from build123d import *

# Parameters (mm, degrees)
SKETCH1_W          = 12.7
SKETCH1_H          = 2.413
CHAMFER1_SIZE      = 0.79375
CUT_EXTRUDE2_DEPTH = 1.79578
SKETCH6_R          = 1.833087105
CUT_EXTRUDE3_DEPTH = 1.79578
CUT_EXTRUDE3_TAPER = 45


with BuildPart() as part:
    # Sketch1 → Revolve1 (revolve)
    with BuildSketch(Plane(origin=(0, 0, 0), x_dir=(0, 0, -1), z_dir=(1, 0, 0))):
        with Locations((8.9154, 1.2065)):
            Rectangle(SKETCH1_W, SKETCH1_H)
    revolve(axis=Axis((0, 0, -15.2654), (0, 0, 1)))

    # Chamfer1
    chamfer1_edges = [part.edges().sort_by_distance(p)[0] for p in [
        (0, -2.413, -15.2654),
    ]]
    chamfer(chamfer1_edges, length=CHAMFER1_SIZE)

    # Sketch7 → Revolve2 (revolve)
    with BuildSketch(Plane(origin=(0, 0, 0), x_dir=(0, 0, -1), z_dir=(1, 0, 0)), mode=Mode.PRIVATE) as revolve2_sk:
        with BuildLine():
            Line((2.18059, 4.5847), (2.5654, 4.5847))
            Line((2.5654, 4.5847), (2.5654, 0))
            Line((2.5654, 0), (0, 0))
            Line((0, 0), (0, 2.413))
            ThreePointArc((0, 2.413), (0.925030326, 3.664791196), (2.18059, 4.5847))
        make_face()
    revolve(revolve2_sk.sketch.rotate(Axis((0, 0, 0), (0, 0, -1)), 180), axis=Axis((0, 0, 0), (0, 0, -1)))

    # Sketch5 → Cut-Extrude2 (cut)
    with BuildSketch(Plane.XY):
        Polygon((1.5875, -0.916543552), (1.5875, 0.916543552), (0, 1.833087105), (-1.5875, 0.916543552), (-1.5875, -0.916543552), (0, -1.833087105), align=None)
    extrude(amount=-CUT_EXTRUDE2_DEPTH, mode=Mode.SUBTRACT)

    # Sketch6 → Cut-Extrude3 (cut)
    with BuildSketch(Plane.XY):
        Circle(SKETCH6_R)
    extrude(amount=-CUT_EXTRUDE3_DEPTH, taper=CUT_EXTRUDE3_TAPER, mode=Mode.SUBTRACT)


solid = part.part
Can you work these out from the model? Positions are in its coordinate system, mm. A direction names the side the tool comes from. Give positions to 0.01 mm unless a question says otherwise; leave off trailing zeros. Loops run counter-clockwise (first coordinate to the right, second up) from the corner with the lowest first, then second, coordinate; pieces in that order, holes last. Notation, with made-up numbers: M 71,-38 L 76,-38 A28 cw 76,-18 Z; hole C 33.5,70.25 d1. An arc over 180 degrees is marked long. One line per item, written item: value.
1) Imagine slicing it at A-A on y = 0. Write out the boundary of the cut face in (x, z).
Geometry check:
outline: M -4.58,-2.57 L -2.41,-2.57 L -2.41,-14.47 L -1.62,-15.27 L 1.62,-15.27 L 2.41,-14.47 L 2.41,-2.57 L 4.58,-2.57 L 4.58,-2.18 A5.17 ccw 2.41,0 L 1.83,0 L 1.59,-0.25 L 1.59,-1.8 L -1.59,-1.8 L -1.59,-0.25 L -1.83,0 L -2.41,0 A5.17 ccw -4.58,-2.18 Z
2) On a 3-axis mill with a long thin cutter (end or side, diameter ignored), from which of +Z, -Z, +X, -X, +Y, -Y can I reach the whole of each face in a straight line? I mean faces 5 (the face through (1.468, -1.915, -8.602)), 6 (the face through (0.865, 1.473, -0.125)), 7 (the face through (-2, 0, 0)). Say none if no direction works.
Geometry check:
face 5: -Z
face 6: +Z
face 7: +Z, +X, -X, +Y, -Y
3) I'm going to push flat-ended pins straight in: pin 1 (1.6 mm diameter, centred on x = 0.5, y = 0.5, fed in from +Z); pin 2 (2 mm diameter, centred on x = -3, z = -7.5, fed in from -Y); pin 3 (1.5 mm diameter, centred on x = -3, y = 2.5, fed in from -Z). Where does each tip first touch, or does it pass through?
Geometry check:
pin 1: stops at z = -1.8
pin 2: stops at y = -1.35
pin 3: stops at z = -2.57
4) Imagine slicing it at B-B on z = -7. Write out the boundary of the cut face in (x, y), and give its area (3 significant figures).
Geometry check:
outline: C 0,0 d4.83
area: 18.3 mm²
5) Thinking about a two-plate mould opening in Y: for faces 1 (the face through (-1.588, 0, -1)), 2 (the face through (-0.783, 1.381, -0.885)), 3 (the face through (4.476, 0.994, -2.376)), 4 (the face through (2, -2, -2.565)), which applies, +Y half, -Y half, draft (parallel to the pull), parting line (faces both ways), or undercut?
Geometry check:
face 1: undercut
face 2: undercut
face 3: parting line
face 4: draft
6) Please list where these lines run through material, in increasing order: line 1 (Z direction, x = 0, y = -0.75); line 2 (Y direction, x = 1, z = -1.5); line 3 (Y direction, x = 1.5, z = -7.75).
Geometry check:
line 1: z = -15.27 to -1.8
line 2: y = -4.04 to -1.26, 1.26 to 4.04
line 3: y = -1.89 to 1.89
7) Imagine slicing it at C-C on x = 3. Write out the boundary of the cut face in (y, z).
Geometry check:
outline: M -3.47,-2.57 L 3.47,-2.57 L 3.47,-2.18 A4.21 ccw -3.47,-2.18 Z
